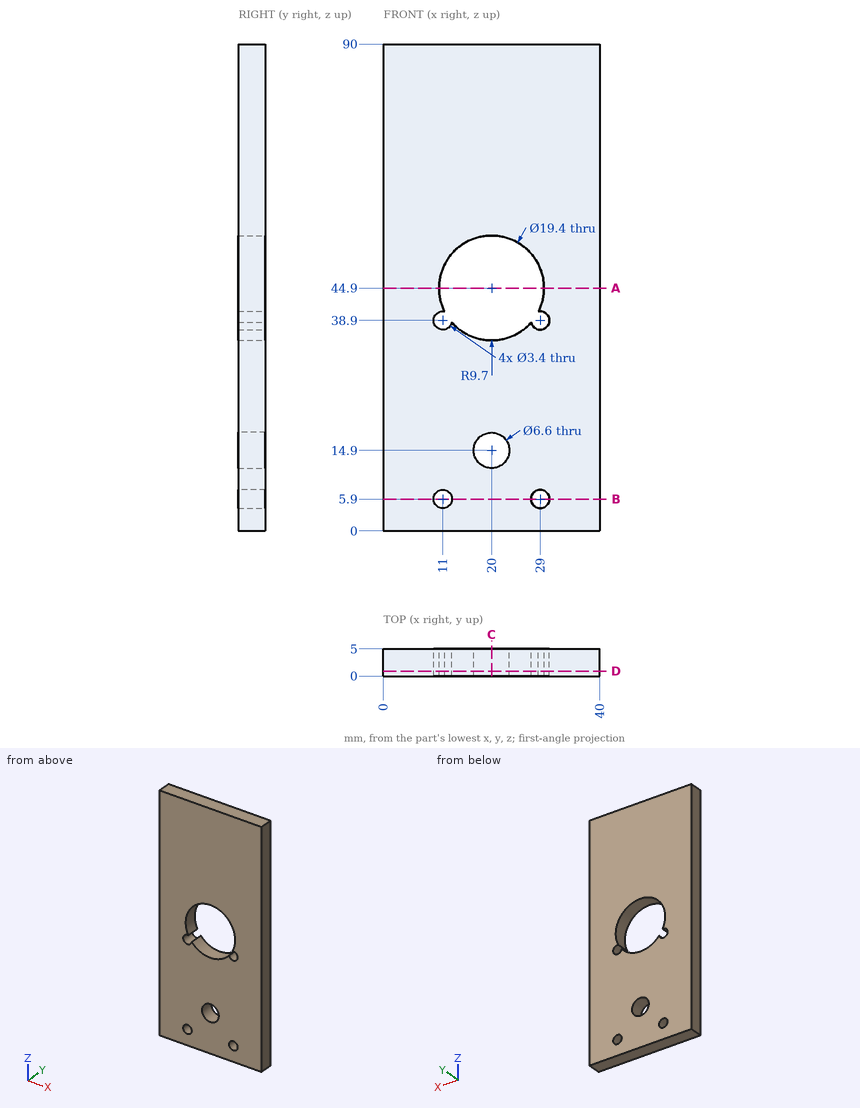
Part print with two shaded views. Sizes in mm from the minimum x, y, z corner. Round coordinates to 2 decimals unless told otherwise and drop trailing zeros. Loops run counter-clockwise (first coordinate to the right, second up) from the corner with the lowest first, then second, coordinate; pieces in that order, holes last. Notation, with made-up numbers: (-26.5, -6) - (5.5, -6) arc R15 cw to (5.5, 17) - close; hole circle Ø3 at (-25, -11.5). An arc over 180 degrees is marked (long way). Put each result on its own line as item: value.
1. Slice it at D-D on y = 0.9. List the corners of the cut face in (x, z).
Geometry check:
outline: (0, 0) - (40, 0) - (40, 90) - (0, 90) - close; hole circle Ø3.4 at (11, 5.9); hole (11.32, 40.57) arc R1.7 ccw (long way) to (12.66, 38.55) arc R9.7 ccw to (27.34, 38.55) arc R1.7 ccw (long way) to (28.68, 40.57) arc R9.7 ccw (long way) to start; hole circle Ø6.6 at (20, 14.9); hole circle Ø3.4 at (29, 5.9)
2. Slice it at C-C on x = 20. List the corners of the cut face in (y, z), and give its area (3 significant figures).
Geometry check:
outline: (0, 0) - (5, 0) - (5, 11.6) - (0, 11.6) - close; (0, 18.2) - (5, 18.2) - (5, 35.2) - (0, 35.2) - close; (0, 54.6) - (5, 54.6) - (5, 90) - (0, 90) - close
area: 320 mm²
3. Pin check, flat tips, straight feed: P1, Ø1.5, axis at x = 27, y = 2, coming from the -Z side; P2, Ø2.5, axis at x = 11, z = 38.9, coming from the -Y side. Stop position of each tip, or through.
Geometry check:
P1: z = 0
P2: through
4. Slice it at A-A on z = 44.9. List the corners of the cut face in (x, y), and give its area (3 significant figures).
Geometry check:
outline: (0, 0) - (10.3, 0) - (10.3, 5) - (0, 5) - close; (29.7, 0) - (40, 0) - (40, 5) - (29.7, 5) - close
area: 103 mm²
5. Wall check: line 1 (X direction, y = 3.1, z = 5.9); line 2 (Z direction, x = 29, y = 2.3); line 3 (Z direction, x = 28, y = 1.85). Give the ranges that are in metal, low to high.
Geometry check:
line 1: 0 to 9.3, 12.7 to 27.3, 30.7 to 40
line 2: 0 to 4.2, 7.6 to 37.2, 40.6 to 41.28, 48.52 to 90
line 3: 0 to 4.53, 7.27 to 37.53, 50.39 to 90
6. Slice it at B-B on z = 5.9. List the corners of the cut face in (x, y).
Geometry check:
outline: (0, 0) - (9.3, 0) - (9.3, 5) - (0, 5) - close; (12.7, 0) - (27.3, 0) - (27.3, 5) - (12.7, 5) - close; (30.7, 0) - (40, 0) - (40, 5) - (30.7, 5) - close
